Check sheet for the drawn part. Datum: minimum x, y, z corner. Units: mm. A direction names the side the tool comes from. Give positions to 0.01 mm unless a question says otherwise; leave off trailing zeros. Loops run counter-clockwise (first coordinate to the right, second up) from the corner with the lowest first, then second, coordinate; pieces in that order, holes last. Notation, with made-up numbers: (44.5, 42) - (92.5, 42) arc R23 ccw to (92.5, 59) - close; hole circle Ø10 at (3.25, 71.5). An arc over 180 degrees is marked (long way). Answer in a Markdown table with one row per item.
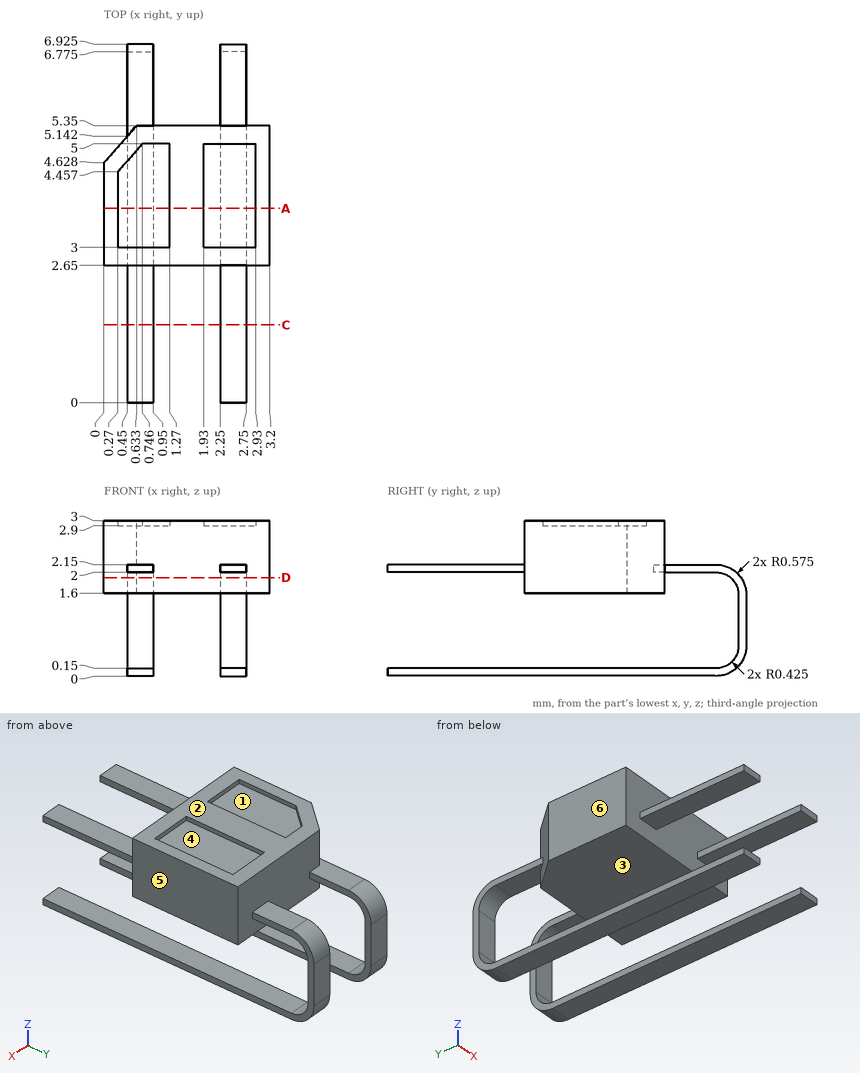
Q1. Sectioned sample at A-A (y = 3.75). Record the cut outline in (x, z).
Completed:
| item | result |
|---|---|
| outline | (0, 1.6) - (3.2, 1.6) - (3.2, 3) - (2.93, 3) - (2.93, 2.9) - (1.93, 2.9) - (1.93, 3) - (1.27, 3) - (1.27, 2.9) - (0.27, 2.9) - (0.27, 3) - (0, 3) - close; (0.45, 0) - (0.95, 0) - (0.95, 0.15) - (0.45, 0.15) - close; (2.25, 0) - (2.75, 0) - (2.75, 0.15) - (2.25, 0.15) - close |
Q2. Sectioned sample at D-D (z = 1.9). Give the number of separate pieces and of enclosed holes in the cut face.
Completed:
| item | result |
|---|---|
| separate pieces | 3 |
| enclosed holes | 0 |
Q3. Draft check along X on the marked faces 4, 5 and 6. Enter one of: +X half, -X half, draft (parallel to the pull), parting line (faces both ways), or undercut.
Completed:
| item | result |
|---|---|
| face 4 | undercut |
| face 5 | +X half |
| face 6 | -X half |
Q4. Sectioned sample at C-C (y = 1.5). Record the cut outline in (x, z).
Completed:
| item | result |
|---|---|
| outline | (0.45, 0) - (0.95, 0) - (0.95, 0.15) - (0.45, 0.15) - close; (0.45, 2) - (0.95, 2) - (0.95, 2.15) - (0.45, 2.15) - close; (2.25, 0) - (2.75, 0) - (2.75, 0.15) - (2.25, 0.15) - close; (2.25, 2) - (2.75, 2) - (2.75, 2.15) - (2.25, 2.15) - close |
Q5. Go/stop test with a flat-tipped pin: P1, Ø0.7, axis at x = 2, z = 2.5, coming from the +Y side. Record where the tip stops, or that it passes through.
Completed:
| item | result |
|---|---|
| P1 | y = 5.35 |
Q6. Tool access check on the marked faces 1, 2 and 3. Record the directions out of +Z, -Z, +X, -X, +Y, -Y that give a thin tool (end or side, any length) a straight path to the whole face; none if there is none.
Completed:
| item | result |
|---|---|
| face 1 | +Z |
| face 2 | +Z, +X, -X, +Y, -Y |
| face 3 | +X, -X, -Y |
Q7. Thickness scan on line 1 (Z direction, x = 0.6, y = 4.5); line 2 (Z direction, x = 1.1, y = 5.25); line 3 (Y direction, x = 2.35, z = 2.7). Record the ranges inside material, lowest first.
Completed:
| item | result |
|---|---|
| line 1 | 0 to 0.15, 1.6 to 2.9 |
| line 2 | 1.6 to 3 |
| line 3 | 2.65 to 5.35 |
